For this review, take the finished solid that the model builds, in its own axes (mm). A direction names the side the tool comes from. Give positions to 0.01 mm unless a question says otherwise; leave off trailing zeros. Loops run counter-clockwise (first coordinate to the right, second up) from the corner with the lowest first, then second, coordinate; pieces in that order, holes last.
Autodesk Inventor part; units mm, degrees
ref_plane "YZ Plane" through (0, 0, 0) normal (1, 0, 0) x (0, 1, 0)
ref_plane "XZ Plane" through (0, 0, 0) normal (0, 1, 0) x (-1, 0, 0)
ref_plane "XY Plane" through (0, 0, 0) normal (0, 0, 1) x (1, 0, 0)
sketch "Sketch1" plane through (0, 0, 0) normal (1, 0, 0) x (0, 1, 0)
  line L0 (4.05, 4.05) -> (-4.05, 4.05)
  line L1 (-4.05, 4.05) -> (-4.05, -4.05)
  line L2 (-4.05, -4.05) -> (4.05, -4.05)
  line L3 (4.05, -4.05) -> (4.05, 4.05)
  line L4 (11.55, 15) -> (4.05, 15)
  line L5 (4.05, 15) -> (4.05, -15)
  line L6 (4.05, -15) -> (11.55, -15)
  line L7 (11.55, -15) -> (11.55, 15)
  line L8 (4.05, 4.05) -> (-4.05, -4.05) construction
  line L9 (4.05, -4.05) -> (-4.05, 4.05) construction
  line L10 (2.05, 2.05) -> (-2.05, 2.05)
  line L11 (-2.05, 2.05) -> (-2.05, -2.05)
  line L12 (-2.05, -2.05) -> (2.05, -2.05)
  line L13 (2.05, -2.05) -> (2.05, 2.05)
  line L14 (2.05, 2.05) -> (-2.05, -2.05) construction
  line L15 (-2.05, 2.05) -> (2.05, -2.05) construction
  point P0 (4.05, 4.05)
  point P1 (0, 0)
  point P2 (0, 0)
  point P3 (0, 0)
  dimension "d0" = 8.1
  dimension "d3" = 8.1
  dimension "d22" = 10.95
  dimension "d24" = 30
  dimension "d25" = 7.5
  dimension "d55" = 10.95
  dimension "d65" = 4.1
  dimension "d66" = 4.1
extrude "Extrusion1" add sketch "Sketch1" along normal blind 15
sketch "Sketch5" plane through (0, 4.05, 15) normal (0, 0, 1) x (1, 0, 0)
  line L0 (7.15, 5.25) -> (7.85, 5.25)
  line L1 (7.85, 5.25) -> (7.85, 2.25)
  line L2 (7.85, 2.25) -> (7.15, 2.25)
  line L3 (7.15, 2.25) -> (7.15, 5.25)
  line L4 (0, 0) -> (15, 0)
  line L5 (0, 7.5) -> (0, 0)
  point P0 (0, -4.05)
  dimension "d86" = 3
  dimension "d87" = 0.7
  dimension "d88" = 2.25
  dimension "d89" = 7.15
extrude "Extrusion4" cut sketch "Sketch5" against normal through all
fillet "Fillet3" radius 5 2 edges at (7.5, 4.05, 4.05) (7.5, 4.05, -4.05)
sketch "Sketch7" plane through (0, 0, 0) normal (-1, 0, 0) x (0, 0, 1)
  line L0 (3.7, 11.55) -> (1.7, 11.55)
  line L1 (1.7, 11.55) -> (1.7, 16.55)
  line L2 (1.7, 16.55) -> (3.7, 16.55)
  line L3 (3.7, 16.55) -> (3.7, 11.55)
  line L4 (3.7, 11.55) -> (1.7, 16.55) construction
  line L5 (1.7, 11.55) -> (3.7, 16.55) construction
  line L6 (-1.7, 11.55) -> (-3.7, 11.55)
  line L7 (-3.7, 11.55) -> (-3.7, 16.55)
  line L8 (-3.7, 16.55) -> (-1.7, 16.55)
  line L9 (-1.7, 16.55) -> (-1.7, 11.55)
  line L10 (-1.7, 11.55) -> (-3.7, 16.55) construction
  line L11 (-3.7, 11.55) -> (-1.7, 16.55) construction
  line L12 (-15, 11.55) -> (15, 11.55)
  point P0 (0, 0)
  point P1 (2.7, 14.05)
  point P2 (-2.7, 14.05)
  dimension "d77" = 5
  dimension "d78" = 2
  dimension "d79" = 2
  dimension "d80" = 3.4
  dimension "d82" = 1.7
extrude "Extrusion5" add sketch "Sketch7" against normal up to surface (15 mm away)
fillet "Fillet4" radius 5 2 edges at (7.5, 11.55, 3.7) (7.5, 11.55, -3.7)
sketch "Sketch8" plane through (0, 11.55, -15) normal (0, 1, 0) x (1, 0, 0)
  line L0 (0, -23.7) -> (15, -23.7)
  line L1 (15, -30) -> (10, -30)
  line L2 (10, -30) -> (10, -23.7)
  line L3 (10, -23.7) -> (15, -23.7)
  line L4 (15, -23.7) -> (15, -30)
  line L5 (0, -30) -> (5, -30)
  line L6 (5, -30) -> (5, -23.7)
  line L7 (5, -23.7) -> (0, -23.7)
  line L8 (0, -23.7) -> (0, -30)
  line L9 (0, -5.95) -> (0, 0)
  line L10 (0, 0) -> (5, 0)
  line L11 (5, 0) -> (5, -6.3)
  line L12 (5, -6.3) -> (0, -6.3)
  line L13 (0, -6.3) -> (0, 0)
  line L14 (15, -6.3) -> (0, -6.3)
  line L15 (15, -5.95) -> (15, 0)
  line L16 (10, -6.3) -> (15, -6.3)
  line L17 (15, -6.3) -> (15, 0)
  line L18 (15, 0) -> (10, 0)
  line L19 (10, 0) -> (10, -6.3)
  point P0 (0, -15)
  dimension "d90" = 5
  dimension "d91" = 5
  dimension "d92" = 5
  dimension "d93" = 5
extrude "Extrusion6" cut sketch "Sketch8" against normal blind 10
fillet "Fillet5" radius 2 4 edges at (5, 7.7939, 8.7) (10, 7.7939, 8.7) (10, 7.7939, -8.7) (5, 7.7939, -8.7)
equation "\"d3\" = d0"
equation "\"d22\" = d55"
properties part number "fuselage_wing_interface_v2" material "ABS Plastic"
Item 1: Tool access review of faces 1 (the flat face through (1, 8, 8.7)), 2 (the flat face through (7, -2, 4.05)), 3 (the flat face through (2, 8, -8.7)), 4 (the flat face through (7, 11.55, 12)): name each direction out of +Z, -Z, +X, -X, +Y, -Y from which nothing blocks a thin tool from reaching the whole face with its end or side.
Answer:
face 1: +Z, -X, +Y, -Y
face 2: +Z, +X, -X, -Y
face 3: -Z, -X, +Y, -Y
face 4: +Z, +X, -X, +Y
Item 2: Clearance check with flat-ended pins moving along their axes: pin 1 Ø1.5 at (x, y) = (8.5, -3) entering from +Z; pin 2 Ø3 at (x, z) = (9.5, 10.5) entering from +Y; pin 3 Ø6 at (x, y) = (11, 0.5) entering from -Z. State where each tip first meets the part, or that it passes through.
Answer:
pin 1: stops at z = 4.05
pin 2: stops at y = 11.55
pin 3: stops at z = -6.77
Item 3: The part is to be moulded in two halves that separate along Y. For faces 5 (the flat face through (7, 4.05, 12)), 6 (the flat face through (7, -2.05, 0)), 7 (the flat face through (0, 6, 0)), say which applies: released by +Y, released by -Y, zero draft, split by the parting line, or undercut.
Answer:
face 5: released by -Y
face 6: undercut
face 7: zero draft
Item 4: Take a section at C-C on y = 8. Give the boundary of the cut face in (x, z), and give its area (3 significant figures).
Answer:
outline: (0, -8.7) - (3, -8.7) arc R2 cw to (5, -10.7) - (5, -15) - (7.15, -15) - (7.15, 15) - (5, 15) - (5, 10.7) arc R2 cw to (3, 8.7) - (0, 8.7) - close; (7.85, -15) - (10, -15) - (10, -10.7) arc R2 cw to (12, -8.7) - (15, -8.7) - (15, 8.7) - (12, 8.7) arc R2 cw to (10, 10.7) - (10, 15) - (7.85, 15) - close
area: 306 mm2
Item 5: For L1, parallel to X at y = 7.5, z = -5.75; L2, parallel to Y at x = 14, z = -2; L3, parallel to Y at x = 4, z = -1.5, list the stretches that pass through material, from the lowest coordinate up.
Answer:
L1: x = 0 to 7.15, 7.85 to 15
L2: y = -4.05 to -2.05, 2.05 to 16.55
L3: y = -4.05 to -2.05, 2.05 to 11.55
Item 6: Take a section at B-B on z = -1. Give the boundary of the cut face in (x, y), and give its area (3 significant figures).
Answer:
outline: (0, -4.05) - (15, -4.05) - (15, -2.05) - (0, -2.05) - close; (0, 2.05) - (15, 2.05) - (15, 11.55) - (0, 11.55) - close; hole (7.15, 6.3) - (7.85, 6.3) - (7.85, 9.3) - (7.15, 9.3) - close
area: 170 mm2
